Input: part model. Units: mm. Frame: model coordinates. A direction names the side the tool comes from. Coordinates: 2 decimals unless noted, no trailing zeros. Write each loop counter-clockwise with the first axis right and the second up, starting at its lowest first coordinate (ties: lowest second). Pieces come first, ordered by that corner, then holes. Notation, with made-up numbers: (59.25, -6) - (94.25, -6) arc R9 cw to (94.25, 6) - close; hole circle Ø2 at (66.25, 7). An arc over 180 degrees is marked (long way). Use CSV: the item, a comma, the result in double quotes.
```python
from build123d import *

# Parameters (mm, degrees)
SKETCH1_W           = 150
SKETCH1_H           = 35
BOSS_EXTRUDE1_DEPTH = 3.18
SKETCH2_R           = 1.55
SKETCH2_W           = 3.18
SKETCH2_H           = 7.625
CUT_EXTRUDE1_DEPTH  = 78.080233523


with BuildPart() as part:
    # Sketch1 → Boss-Extrude1 (new body)
    with BuildSketch(Plane.XY):
        Rectangle(SKETCH1_W, SKETCH1_H)
    extrude(amount=BOSS_EXTRUDE1_DEPTH)

    # Sketch2 → Cut-Extrude1 (cut, through all)
    with BuildSketch(Plane.XY.offset(3.18)):
        with Locations((-73, 0)):
            Circle(SKETCH2_R)
        with Locations((73, 0)):
            Circle(SKETCH2_R)
        Polygon((1.5, 14.32), (10, 14.32), (10, 17.5), (-10, 17.5), (-10, 14.32), (-1.5, 14.32), (-1.5, 10.32), (-3.5, 10.32), (-3.5, 7.32), (-1.5, 7.32), (-1.5, 4.5), (1.5, 4.5), (1.5, 7.32), (3.5, 7.32), (3.5, 10.32), (1.5, 10.32), align=None)
        Polygon((-1.5, -7.32), (-1.5, -4.5), (1.5, -4.5), (1.5, -7.32), (3.5, -7.32), (3.5, -10.32), (1.5, -10.32), (1.5, -14.32), (10, -14.32), (10, -17.5), (-10, -17.5), (-10, -14.32), (-1.5, -14.32), (-1.5, -10.32), (-3.5, -10.32), (-3.5, -7.32), align=None)
        with Locations((73.41, -13.6875)):
            Rectangle(SKETCH2_W, SKETCH2_H)
        with Locations((-73.41, 13.6875)):
            Rectangle(SKETCH2_W, SKETCH2_H)
        with Locations((-73.41, -13.6875)):
            Rectangle(SKETCH2_W, SKETCH2_H)
        with Locations((73.41, 13.6875)):
            Rectangle(SKETCH2_W, SKETCH2_H)
    extrude(amount=-CUT_EXTRUDE1_DEPTH, mode=Mode.SUBTRACT)


solid = part.part
```
(1) Reachability of faces 4 (the flat face through (-1.5, -12, 2)), 5 (the flat face through (-1.5, 6, 2)), 6 (the flat face through (3.5, -9, 2)) from +Z, -Z, +X, -X, +Y, -Y: full face, straight path, thin tool, end or side. Return the list, or none.
Check values:
face 4,"+Z, -Z, -Y"
face 5,"+Z, -Z, +Y"
face 6,"+Z, -Z"
(2) Cut plane A-A on y = -12. Return loops of the section in (x, z).
Check values:
outline,"(-71.82, 0) - (-1.5, 0) - (-1.5, 3.18) - (-71.82, 3.18) - close; (1.5, 0) - (71.82, 0) - (71.82, 3.18) - (1.5, 3.18) - close"
(3) Draft query along X for faces 1 (the flat face through (-75, 0, 2)), 2 (the flat face through (6, 14.32, 2)), 3 (the flat face through (71.82, 14, 2)). Return one class per face: pulls with the +X half, pulls with the -X half, needs draft (parallel to the pull), parting line crosses it, or undercut.
Check values:
face 1,"pulls with the -X half"
face 2,"undercut"
face 3,"pulls with the +X half"
(4) Cut plane B-B on y = 0. Return loops of the section in (x, z).
Check values:
outline,"(-75, 0) - (-74.55, 0) - (-74.55, 3.18) - (-75, 3.18) - close; (-71.45, 0) - (71.45, 0) - (71.45, 3.18) - (-71.45, 3.18) - close; (74.55, 0) - (75, 0) - (75, 3.18) - (74.55, 3.18) - close"
(5) Ray query, probe 1 along Y at (x, z) = (-73, 1.6) (3 decimals); probe 2 along X at (y, z) = (-5, 2.85); probe 3 along X at (y, z) = (16, 2). Return the intervals inside material, ascending. Write a range as from..to.
Check values:
probe 1,"-9.875..-1.55, 1.55..9.875"
probe 2,"-75..-1.5, 1.5..75"
probe 3,"-71.82..-10, 10..71.82"
(6) Cut plane C-C on z = 1. State how many separate pieces and enclosed holes the cut face has, and give its area (3 significant figures).
Check values:
separate pieces,"1"
enclosed holes,"2"
area,"4,930 mm^2"
(7) Pin query (flat end, axial travel): pin 1 Ø1.6 at (x, z) = (2.5, 1) entering from +Y; pin 2 Ø1.5 at (y, z) = (12.5, 1.5) entering from +X; pin 3 Ø0.9 at (x, z) = (0, 2) entering from +Y; pin 4 Ø4 at (x, y) = (-73, 0) entering from +Z. Return the tip coordinate at first contact, or that it passes through.
Check values:
pin 1,"y = 14.32"
pin 2,"x = 71.82"
pin 3,"y = 4.5"
pin 4,"z = 3.18"
(8) Cut plane D-D on x = -7. Return loops of the section in (y, z), and give its area (3 significant figures).
Check values:
outline,"(-14.32, 0) - (14.32, 0) - (14.32, 3.18) - (-14.32, 3.18) - close"
area,"91.1 mm^2"
